```python
from build123d import *

# Parameters (mm, degrees)
F1_DEPTH = 2.5
F3_D     = 11
F3_DEPTH = 24.5
F3_TIP   = 3.3047334047


with BuildPart() as f1:
    # F0 (on Front) → F1 (new body, symmetric)
    with BuildSketch(Plane.XZ):
        with BuildLine():
            Line((40, 103.1), (-40, 103.1))
            ThreePointArc((-40, 103.1), (-47.0710678119, 100.1710678119), (-50, 93.1))
            Line((-50, 93.1), (-50, -93.1))
            ThreePointArc((-50, -93.1), (-47.0710678119, -100.1710678119), (-40, -103.1))
            Line((-40, -103.1), (40, -103.1))
            ThreePointArc((40, -103.1), (47.0710678119, -100.1710678119), (50, -93.1))
            Line((50, -93.1), (50, 93.1))
            ThreePointArc((50, 93.1), (47.0710678119, 100.1710678119), (40, 103.1))
        make_face()
    extrude(amount=F1_DEPTH, both=True)

    # F3
    with Locations(Plane.XZ.offset(2.5)):
        with Locations((-25, 78.1), (25, 78.1), (25, -78.1), (-25, -78.1)):
            Hole(F3_D / 2, depth=F3_DEPTH)
            with Locations((0, 0, -(F3_DEPTH + F3_TIP / 2))):  # 118° drill point
                Cone(0, F3_D / 2, F3_TIP, mode=Mode.SUBTRACT)


solid = f1.part
```
The listing builds one solid part. Answer for the finished solid, in the listing's coordinates (mm). Give positions to 0.01 mm unless a question says otherwise; leave off trailing zeros. Order: outer loops, then holes, each group sorted by start corner. A loop starts at its lowest first (then second) coordinate and runs counter-clockwise, first axis right, second up.
1) Find section A-A on z = 78.1. Write down the section's boundary in (x, y).
Reported:
outline: (-50, -2.5) - (-30.5, -2.5) - (-30.5, 2.5) - (-50, 2.5) - close; (-19.5, -2.5) - (19.5, -2.5) - (19.5, 2.5) - (-19.5, 2.5) - close; (30.5, -2.5) - (50, -2.5) - (50, 2.5) - (30.5, 2.5) - close
2) Determine the mould class of faces 1 (the face through (-50, 0, 1)), 2 (the face through (-23.81, 0.04, -83.47)), 3 (the face through (-47.15, -0.04, -100.09)) for opening direction Z: pulls with the +Z half, pulls with the -Z half, needs draft (parallel to the pull), parting line crosses it, or undercut.
Reported:
face 1: needs draft
face 2: undercut
face 3: pulls with the -Z half
3) Find section B-B on y = -1.55. Write down the section's boundary in (x, z).
Reported:
outline: (-50, -93.1) arc R10 ccw to (-40, -103.1) - (40, -103.1) arc R10 ccw to (50, -93.1) - (50, 93.1) arc R10 ccw to (40, 103.1) - (-40, 103.1) arc R10 ccw to (-50, 93.1) - close; hole circle Ø11 at (-25, -78.1); hole circle Ø11 at (-25, 78.1); hole circle Ø11 at (25, -78.1); hole circle Ø11 at (25, 78.1)
4) Find section C-C on x = -25. Write down the section's boundary in (y, z).
Reported:
outline: (-2.5, -103.1) - (2.5, -103.1) - (2.5, -83.6) - (-2.5, -83.6) - close; (-2.5, -72.6) - (2.5, -72.6) - (2.5, 72.6) - (-2.5, 72.6) - close; (-2.5, 83.6) - (2.5, 83.6) - (2.5, 103.1) - (-2.5, 103.1) - close
5) Consider line 1 along Z through (x, y) = (-25, -0.45); line 2 along Z through (x, y) = (-21.5, 0.6); line 3 along Z through (x, y) = (40.5, -2.25). Determine where each line is inside the solid, lowest interval first.
Reported:
line 1: z = -103.1 to -83.6, -72.6 to 72.6, 83.6 to 103.1
line 2: z = -103.1 to -82.34, -73.86 to 73.86, 82.34 to 103.1
line 3: z = -103.09 to 103.09
